Could you check a few things on this model? Use its own coordinates, in mm. A direction names the side the tool comes from. Coordinates: 2 decimals unless noted, no trailing zeros. Loops run counter-clockwise (first coordinate to the right, second up) from the corner with the lowest first, then second, coordinate; pieces in that order, holes last.
1) Imagine slicing it at C-C on x = -71. Please give me the cut outline in (y, z), plus the area to 3 significant figures.
2) If I drill on line 1 along X through (y, z) = (-9, 72); line 2 along X through (y, z) = (-0.25, -31.5); line 3 along Z through (x, y) = (-70.5, -11.5), over which ranges is the centre line in solid material (lowest first)?
3) Will these pins go through, and if not, where does the flat tip stop? P1, Ø3.5, axis at y = -3, z = 38.5, coming from the +X side; P2, Ø1, axis at x = -14, y = -3, coming from the +Z side; P3, Ø6, axis at y = -5.5, z = 26.5, coming from the -X side; P4, Ø8, axis at y = -3, z = -19, coming from the +X side.
4) Imagine slicing it at A-A on x = 87.5. Please give me the cut outline in (y, z).
5) Thinking about a two-plate mould opening in Z: for faces 1 (the face through (101.99, 1.01, -102.15)), 2 (the face through (-83, -4, 23)), 3 (the face through (-25, 2, -48)), which applies, released by +Z, released by -Z, zero draft, split by the parting line, or undercut?
6) For faces 4 (the face through (11, -6, -28)), 5 (the face through (-14.25, -4, 66)), 6 (the face through (-15, -6, -14)), which set-ups out of +Z, -Z, +X, -X, +Y, -Y let a thin tool reach every point of the face, with its end or its side?
7) Imagine slicing it at D-D on z = -21.5. Please give me the cut outline in (x, y), plus the area to 3 significant figures.
8) Imagine slicing it at B-B on z = 30. Please give me the cut outline in (x, y).
```python
from build123d import *

# Parameters (mm, degrees)
SKETCH1_W           = 210
SKETCH1_H           = 210
MAINEXTRUDE_DEPTH   = 2
SKETCH1_6_R         = 1.5
SCREWHOLES_DEPTH    = 2
ROUNDEDCORNERS_R    = 10
TRENCH_DEPTH        = 12
BOSS_EXTRUDE3_DEPTH = 10
BOSS_EXTRUDE4_DEPTH = 2


with BuildPart() as part:
    # Sketch1 → MainExtrude (new body)
    with BuildSketch(Plane(origin=(0, 0, 0), x_dir=(1, 0, 0), z_dir=(0, 1, 0))):
        Rectangle(SKETCH1_W, SKETCH1_H)
    extrude(amount=MAINEXTRUDE_DEPTH)

    # Sketch1<6> → ScrewHoles (cut)
    with BuildSketch(Plane(origin=(0, 0, 0), x_dir=(1, 0, 0), z_dir=(0, 1, 0))):
        with Locations((-99.833273811, 99.833273811)):
            Circle(SKETCH1_6_R)
        with Locations((-99.833273811, -99.833273811)):
            Circle(SKETCH1_6_R)
        with Locations((99.833273811, -99.833273811)):
            Circle(SKETCH1_6_R)
        with Locations((99.833273811, 99.833273811)):
            Circle(SKETCH1_6_R)
    extrude(amount=SCREWHOLES_DEPTH, mode=Mode.SUBTRACT)

    # RoundedCorners
    roundedcorners_edges = [part.edges().sort_by_distance(p)[0] for p in [
        (-105, 1, -105),
        (-105, 1, 105),
        (105, 1, 105),
        (105, 1, -105),
    ]]
    fillet(roundedcorners_edges, radius=ROUNDEDCORNERS_R)

    # Sketch3 → Trench (cut)
    with BuildSketch(Plane(origin=(0, 0, 0), x_dir=(1, 0, 0), z_dir=(0, 1, 0))):
        Polygon((-64.25, 93), (-64.25, 26), (-93, 26), (-93, 16), (64.5, 16), (64.5, -39.5), (-83, -39.5), (-83, -6), (41, -6), (41, 4), (-93, 4), (-93, -49.5), (-24.25, -49.5), (-24.25, -93), (93, -93), (93, 94.5), (-24.25, 94.5), (-24.25, 84.5), (83, 84.5), (83, -83), (-14.25, -83), (-14.25, -49.5), (74.5, -49.5), (74.5, 26), (-54.25, 26), (-54.25, 93), align=None)
    extrude(amount=TRENCH_DEPTH, mode=Mode.SUBTRACT)

    # Sketch7 → Boss-Extrude3 (add)
    with BuildSketch(Plane.XZ):
        Polygon((-66.25, -95), (-52.25, -95), (-52.25, -28), (76.5, -28), (76.5, 51.5), (-12.25, 51.5), (-12.25, 81), (81, 81), (81, -82.5), (-26.25, -82.5), (-26.25, -96.5), (95, -96.5), (95, 95), (-26.25, 95), (-26.25, 51.5), (-95, 51.5), (-95, -6), (43, -6), (43, 8), (-81, 8), (-81, 37.5), (62.5, 37.5), (62.5, -14), (-95, -14), (-95, -28), (-66.25, -28), align=None)
        Polygon((-64.25, -93), (-54.25, -93), (-54.25, -26), (74.5, -26), (74.5, 49.5), (-14.25, 49.5), (-14.25, 83), (83, 83), (83, -84.5), (-24.25, -84.5), (-24.25, -94.5), (93, -94.5), (93, 93), (-24.25, 93), (-24.25, 49.5), (-93, 49.5), (-93, -4), (41, -4), (41, 6), (-83, 6), (-83, 39.5), (64.5, 39.5), (64.5, -16), (-93, -16), (-93, -26), (-64.25, -26), align=None, mode=Mode.SUBTRACT)
    extrude(amount=BOSS_EXTRUDE3_DEPTH)

    # Sketch8 → Boss-Extrude4 (add)
    with BuildSketch(Plane.XZ.offset(10)):
        Polygon((-66.25, -28), (-66.25, -95), (-52.25, -95), (-52.25, -28), (76.5, -28), (76.5, 51.5), (-12.25, 51.5), (-12.25, 81), (81, 81), (81, -82.5), (-26.25, -82.5), (-26.25, -96.5), (95, -96.5), (95, 95), (-26.25, 95), (-26.25, 51.5), (-95, 51.5), (-95, -6), (43, -6), (43, 8), (-81, 8), (-81, 37.5), (62.5, 37.5), (62.5, -14), (-95, -14), (-95, -28), align=None)
    extrude(amount=BOSS_EXTRUDE4_DEPTH)


solid = part.part
```
Filled in:
1. outline: (-12, -28) - (0, -28) - (0, -105) - (2, -105) - (2, -26) - (-10, -26) - (-10, -16) - (2, -16) - (2, -4) - (-10, -4) - (-10, 6) - (2, 6) - (2, 39.5) - (-10, 39.5) - (-10, 49.5) - (2, 49.5) - (2, 105) - (0, 105) - (0, 51.5) - (-12, 51.5) - (-12, 37.5) - (0, 37.5) - (0, 8) - (-12, 8) - (-12, -6) - (0, -6) - (0, -14) - (-12, -14) - close
1. area: 564 mm2
2. line 1: x = -26.25 to -24.25, -14.25 to -12.25, 81 to 83, 93 to 95
2. line 2: x = -66.25 to -64.25, -54.25 to -52.25, 81 to 83, 93 to 95
2. line 3: z = -28 to -14, -6 to 8, 37.5 to 51.5
3. P1: stops at x = 95
3. P2: stops at z = 95
3. P3: stops at x = -95
3. P4: stops at x = 105
4. outline: (-12, -96.5) - (0, -96.5) - (0, -105) - (2, -105) - (2, -94.5) - (-10, -94.5) - (-10, 93) - (2, 93) - (2, 105) - (0, 105) - (0, 95) - (-12, 95) - close
5. face 1: released by -Z
5. face 2: undercut
5. face 3: zero draft
6. face 4: -Y
6. face 5: +Y
6. face 6: -X, -Y
7. outline: (-105, 0) - (-95, 0) - (-95, -12) - (76.5, -12) - (76.5, 0) - (81, 0) - (81, -12) - (95, -12) - (95, 0) - (105, 0) - (105, 2) - (93, 2) - (93, -10) - (83, -10) - (83, 2) - (74.5, 2) - (74.5, -10) - (-93, -10) - (-93, 2) - (-105, 2) - close
7. area: 516 mm2
8. outline: (-105, 0) - (-95, 0) - (-95, -12) - (-81, -12) - (-81, 0) - (62.5, 0) - (62.5, -12) - (76.5, -12) - (76.5, 0) - (81, 0) - (81, -12) - (95, -12) - (95, 0) - (105, 0) - (105, 2) - (93, 2) - (93, -10) - (83, -10) - (83, 2) - (74.5, 2) - (74.5, -10) - (64.5, -10) - (64.5, 2) - (-83, 2) - (-83, -10) - (-93, -10) - (-93, 2) - (-105, 2) - close
